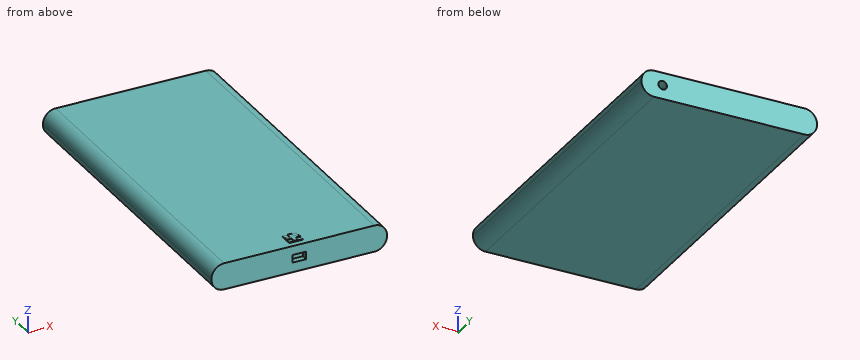
from build123d import *

# Parameters (mm, degrees)
F0_W      = 70.866
F0_H      = 130.302
F1_DEPTH  = 10.668
F2_R      = 5.08
F3_W      = 3.556
F3_H      = 3.128736
F4_DEPTH  = 2.54
F4_FACE_W = 2.54
F4_FACE_H = 3.128736
F5_DEPTH  = 2.053641
F6_R      = 1.75
F7_DEPTH  = 5.334
F8_W      = 1.8695
F8_H      = 3.128736
F9_DEPTH  = 2.54
F10_W     = 1.905
F10_H     = 1.905
F11_DEPTH = 0.254
F12_DEPTH = 0.4826


with BuildPart() as f1:
    # F0 (on Top) → F1 (new body)
    with BuildSketch(Plane.XY):
        with Locations((-48.638468, -11.206365)):
            Rectangle(F0_W, F0_H)
    extrude(amount=F1_DEPTH)

    # F2
    f2_edges = [f1.edges().sort_by_distance(p)[0] for p in [
        (-13.205468, -11.206365, 10.668),
        (-13.205468, -11.206365, 0),
        (-84.071468, -11.206365, 0),
        (-84.071468, -11.206365, 10.668),
    ]]
    fillet(f2_edges, radius=F2_R)

    # F3 (on face) → F4 (cut)
    with BuildSketch(Plane.XZ.offset(76.357365)):
        with Locations((-51.39454, 5.471042)):
            Rectangle(F3_W, F3_H)
        with Locations((-45.784899, 5.471042)):
            Rectangle(F3_W, F3_H)
    extrude(amount=-F4_DEPTH, mode=Mode.SUBTRACT)

    # F4_face (on face) → F5 (cut, through all)
    with BuildSketch(Plane(origin=(-47.562899, -75.087365, 5.471042), x_dir=(0, 1, 0), z_dir=(1, 0, 0))):
        Rectangle(F4_FACE_W, F4_FACE_H)
    extrude(amount=-F5_DEPTH, mode=Mode.SUBTRACT)

    # F6 (on face) → F7 (cut)
    with BuildSketch(Plane(origin=(0, 53.944635, 0), x_dir=(-1, 0, 0), z_dir=(0, 1, 0))):
        with Locations((21.710483, 5.5652)):
            Circle(F6_R)
    extrude(amount=-F7_DEPTH, mode=Mode.SUBTRACT)

    # F8 (on face) → F9 (join, through all)
    with BuildSketch(Plane.XZ.offset(73.817365)):
        with Locations((-52.23779, 5.471042)):
            Rectangle(F8_W, F8_H)
        with Locations((-44.941649, 5.471042)):
            Rectangle(F8_W, F8_H)
    extrude(amount=F9_DEPTH)

    # F10 (on face) → F11 (join)
    with BuildSketch(Plane.XY.offset(10.668)):
        with Locations((-50.41425, -69.658694)):
            Rectangle(F10_W, F10_H)
        with Locations((-50.41425, -72.896037)):
            Rectangle(F10_W, F10_H)
        with Locations((-46.862685, -72.896037)):
            Rectangle(F10_W, F10_H)
        with Locations((-46.862685, -69.658694)):
            Rectangle(F10_W, F10_H)
    extrude(amount=F11_DEPTH)

    # F10 (on face) → F12 (join)
    with BuildSketch(Plane.XY.offset(10.668)):
        Polygon((-49.46175, -68.706194), (-49.46175, -70.611194), (-51.36675, -70.611194), (-51.36675, -71.943537), (-49.46175, -71.943537), (-49.46175, -73.848537), (-47.815185, -73.848537), (-47.815185, -71.943537), (-45.910185, -71.943537), (-45.910185, -70.611194), (-47.815185, -70.611194), (-47.815185, -68.706194), align=None)
    extrude(amount=F12_DEPTH)


solid = f1.part
Work out the finished part from the listing and answer in its coordinate system (mm). Coordinates: 2 decimals unless noted, no trailing zeros. Write each loop counter-clockwise with the first axis right and the second up, starting at its lowest first coordinate (ties: lowest second). Pieces come first, ordered by that corner, then holes. Notation, with made-up numbers: M -23,-27 L 25,-27 A30 ccw 25,1 Z; hole C -2.75,-9 d5. An arc over 180 degrees is marked long. Answer as CSV lines item,"result". Start each with the question number.
Item 1: Section C-C on z = 1.5 is taken. Write down the section's boundary in (x, y), and give its area (3 significant figures).
Item 2: Section B-B on x = -26.5 is taken. Write down the section's boundary in (y, z).
Item 3: Consider L1, parallel to Z at x = -19.5, y = -70; L2, parallel to Y at x = -49, z = 4.5; L3, parallel to X at y = -53.5, z = 6. Determine where each line is inside the solid, lowest interval first.
Item 4: Section A-A on y = 18.5 is taken. Write down the section's boundary in (x, z).
Item 5: Flat-ended cylindrical pins translate along their axes: P1, Ø12, axis at x = -62.5, y = -59, coming from the +Z side; P2, Ø0.6, axis at x = -47, y = -69.5, coming from the +Z side; P3, Ø3, axis at x = -21.71, z = 5.57, coming from the +Y side. Find the tip coordinate at first contact, or state that the pin passes through.
Checks:
1,outline,"M -82.6,-76.36 L -14.68,-76.36 L -14.68,53.94 L -82.6,53.94 Z"
1,area,"8,850 mm²"
2,outline,"M -76.36,0 L 53.94,0 L 53.94,10.67 L -76.36,10.67 Z"
3,L1,"z = 0 to 10.67"
3,L2,"y = -73.82 to 53.94"
3,L3,"x = -84.05 to -13.22"
4,outline,"M -84.07,5.08 A5.08 ccw -78.99,0 L -18.29,0 A5.08 ccw -13.21,5.08 L -13.21,5.59 A5.08 ccw -18.29,10.67 L -78.99,10.67 A5.08 ccw -84.07,5.59 Z"
5,P1,"stops at z = 10.67"
5,P2,"stops at z = 10.92"
5,P3,"stops at y = 48.61"
